Can you work these out from the model? Positions are in its coordinate system, mm. Face numbers are marked on the shaded views. A direction names the side the tool comes from. Give positions to 0.01 mm unless a question says otherwise; leave off trailing zeros. Loops run counter-clockwise (first coordinate to the right, second up) from the corner with the lowest first, then second, coordinate; pieces in that order, holes last. Notation, with made-up numbers: (84, -26.75) -> (100, -26.75) arc R20 ccw to (100, -1.75) -> close; hole circle Ø2 at (19, 30.5). An arc over 180 degrees is marked (long way). Use CSV: the item, a comma, the result in double quotes.
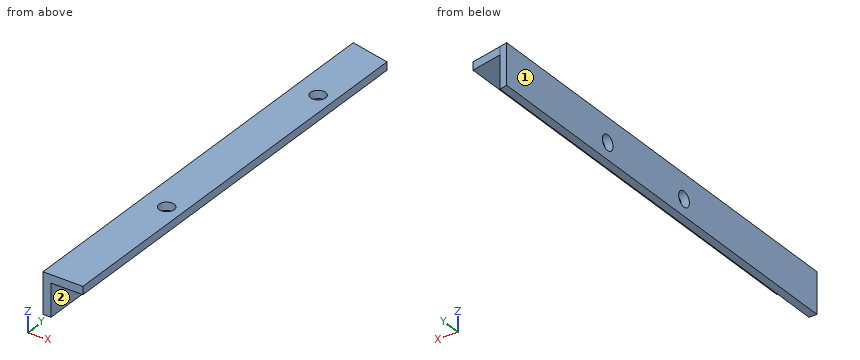
from build123d import *

# Parameters (mm, degrees)
BOSS_EXTRUDE1_DEPTH     = 140
CUT_EXTRUDE1_DEPTH      = 18.35
CUT_EXTRUDE1_DEPTH_BACK = 6.35
SKETCH3_R               = 2.415
CUT_EXTRUDE2_DEPTH      = 10
SKETCH4_R               = 2.415
CUT_EXTRUDE3_DEPTH      = 10
SKETCH5_R               = 2.415
CUT_EXTRUDE4_DEPTH      = 10
SKETCH6_R               = 2.415
CUT_EXTRUDE5_DEPTH      = 10


with BuildPart() as part:
    # Sketch1 → Boss-Extrude1 (new body)
    with BuildSketch(Plane(origin=(0, 0, 0), x_dir=(1, 0, 0), z_dir=(0, 1, 0))):
        Polygon((0, 0), (0, 12.99972), (2.54, 12.99972), (2.54, 2.54), (12.7, 2.54), (12.7, 0), align=None)
    extrude(amount=BOSS_EXTRUDE1_DEPTH)

    # Sketch2 → Cut-Extrude1 (cut, two sides)
    with BuildSketch(Plane(origin=(0, 0, -2.54), x_dir=(-1, 0, 0), z_dir=(0, 0, -1))) as cut_extrude1_sk:
        Polygon((-2.54, 139.443868054), (0, 140), (-11.159733345, 144.634657465), (-16.37733561, 136.414189162), (-12.7, 137.219340268), (-12.7, 140), (-2.54, 140), align=None)
        Polygon((-12.7, 137.219340268), (-2.54, 139.443868054), (-2.54, 140), (-12.7, 140), align=None)
    extrude(amount=CUT_EXTRUDE1_DEPTH, mode=Mode.SUBTRACT)
    extrude(cut_extrude1_sk.sketch, amount=-CUT_EXTRUDE1_DEPTH_BACK, mode=Mode.SUBTRACT)

    # Sketch3 → Cut-Extrude2 (cut)
    with BuildSketch(Plane(origin=(0, 0, -2.54), x_dir=(-1, 0, 0), z_dir=(0, 0, -1))):
        with Locations((-7.62, 113.331604161)):
            Circle(SKETCH3_R)
    extrude(amount=-CUT_EXTRUDE2_DEPTH, mode=Mode.SUBTRACT)

    # Sketch4 → Cut-Extrude3 (cut)
    with BuildSketch(Plane(origin=(2.54, 0, 0), x_dir=(0, 0, -1), z_dir=(1, 0, 0))):
        with Locations((7.76986, 94.443868054)):
            Circle(SKETCH4_R)
    extrude(amount=-CUT_EXTRUDE3_DEPTH, mode=Mode.SUBTRACT)

    # Sketch5 → Cut-Extrude4 (cut)
    with BuildSketch(Plane(origin=(2.54, 0, 0), x_dir=(0, 0, -1), z_dir=(1, 0, 0))):
        with Locations((7.76986, 60)):
            Circle(SKETCH5_R)
    extrude(amount=-CUT_EXTRUDE4_DEPTH, mode=Mode.SUBTRACT)

    # Sketch6 → Cut-Extrude5 (cut)
    with BuildSketch(Plane(origin=(0, 0, -2.54), x_dir=(-1, 0, 0), z_dir=(0, 0, -1))):
        with Locations((-7.62, 45)):
            Circle(SKETCH6_R)
    extrude(amount=-CUT_EXTRUDE5_DEPTH, mode=Mode.SUBTRACT)


solid = part.part
(1) Will these pins go through, and if not, where does the flat tip stop? pin 1 Ø1 at (y, z) = (106.5, -6) entering from -X; pin 2 Ø5.5 at (y, z) = (60, -7.77) entering from +X.
Answer sheet:
pin 1,"stops at x = 0"
pin 2,"stops at x = 2.54"
(2) If we section it at D-D, the plane y = 10.5: Write out the boundary of the cut face in (x, z), then the cut area to 3 significant figures.
Answer sheet:
outline,"(0, -13) -> (2.54, -13) -> (2.54, -2.54) -> (12.7, -2.54) -> (12.7, 0) -> (0, 0) -> close"
area,"58.8 mm2"
(3) If we section it at A-A, the plane y = 45: Write out the boundary of the cut face in (x, z) (3 decimals).
Answer sheet:
outline,"(0, -13) -> (2.54, -13) -> (2.54, -2.54) -> (5.205, -2.54) -> (5.205, 0) -> (0, 0) -> close; (10.035, -2.54) -> (12.7, -2.54) -> (12.7, 0) -> (10.035, 0) -> close"
(4) Which directions (+Z, -Z, +X, -X, +Y, -Y) give clear straight access to the entire face, cutting with the end or side of a thin tool? Please do the marked faces 1 and 2.
Answer sheet:
face 1,"+Z, -Z, -X, +Y, -Y"
face 2,"-Z, +X, +Y, -Y"
(5) If we section it at B-B, the plane x = 8.5: Write out the boundary of the cut face in (y, z), then the cut area to 3 significant figures.
Answer sheet:
outline,"(0, -2.54) -> (42.75, -2.54) -> (42.75, 0) -> (0, 0) -> close; (47.25, -2.54) -> (111.08, -2.54) -> (111.08, 0) -> (47.25, 0) -> close; (115.58, -2.54) -> (138.14, -2.54) -> (138.14, 0) -> (115.58, 0) -> close"
area,"328 mm2"
(6) If I drill on L1, parallel to Y at x = 7.62, z = -1 (3 decimals); L2, parallel to Y at x = 0.5, z = -9.5; L3, parallel to X at y = 65, z = -10.75, over which ranges is the centre line in solid material (lowest first)? Write a range as from..to.
Answer sheet:
L1,"y = 0..42.585, 47.415..110.917, 115.747..138.332"
L2,"y = 0..58.32, 61.68..92.76, 96.13..139.89"
L3,"x = 0..2.54"
(7) If we section it at C-C, the plane z = -6.75: Write out the boundary of the cut face in (x, y), then the cut area to 3 significant figures.
Answer sheet:
outline,"(0, 0) -> (2.54, 0) -> (2.54, 57.81) -> (0, 57.81) -> close; (0, 62.19) -> (2.54, 62.19) -> (2.54, 92.25) -> (0, 92.25) -> close; (0, 96.63) -> (2.54, 96.63) -> (2.54, 139.44) -> (0, 140) -> close"
area,"333 mm2"
